Here's how the part is built. I have some questions about the finished solid (model axes, mm). Face numbers are marked on the shaded views. A direction names the side the tool comes from. Coordinates: 2 decimals unless noted, no trailing zeros. Loops run counter-clockwise (first coordinate to the right, second up) from the corner with the lowest first, then second, coordinate; pieces in that order, holes last. Notation, with made-up numbers: M 78.5,-29 L 109.5,-29 A28 ccw 109.5,-2 Z; hole C 25.5,-18.5 d3. An arc over 180 degrees is marked long. Use one line per item in the form item = value. Start each with the question number.
(1) Will these pins go through, and if not, where does the flat tip stop? P1, Ø6, axis at x = 18.5, z = 10.5, coming from the -Y side; P2, Ø2, axis at y = -5.5, z = 6.5, coming from the +X side; P3, Ø10, axis at x = 16.5, z = 9, coming from the +Y side.
(2) Imagine slicing it at A-A, the plane z = 10.25. Please give me the cut outline in (x, y).
(3) Please list where these lines run through material, in increasing order: L1, parallel to Y at x = 14, z = 13; L2, parallel to Z at x = 42, y = 3.5; L3, parallel to Z at x = 49.5, y = -3.75.
(4) Imagine slicing it at C-C, the plane x = 16.5. Please give me the cut outline in (y, z), and give its area (3 significant figures).
(5) Imagine slicing it at D-D, the plane z = 18.75. Please give me the cut outline in (x, y).
(6) On a 3-axis mill with a long thin cutter (end or side, diameter ignored), from which of +Z, -Z, +X, -X, +Y, -Y can I reach the whole of each face in a straight line? I mean the marked faces 1, 2, 3, 4 and 5. Say none if no direction works.
(7) Imagine slicing it at B-B, the plane y = 2.75. Please give me the cut outline in (x, z), and give its area (3 significant figures).
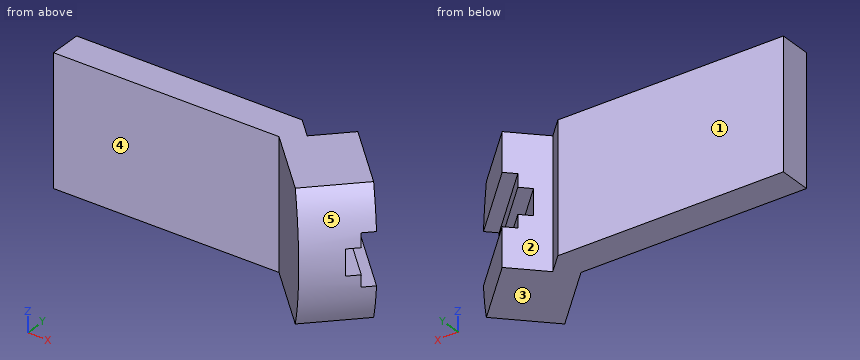
```python
from build123d import *

# Parameters (mm, degrees)
BOSS_EXTRUDE1_DEPTH      = 20
CUT_EXTRUDE5_DEPTH       = 6
CUT_EXTRUDE5_DEPTH_BACK  = 45.944197614
CUT_EXTRUDE10_DEPTH      = 8.5
CUT_EXTRUDE10_DEPTH_BACK = 43.444197614


with BuildPart() as part:
    # Sketch2 → Boss-Extrude1 (new body)
    with BuildSketch(Plane.XY):
        Polygon((0, 0), (35, 0), (45.883024287, -10.883024287), (52.954092099, -3.811956475), (42.347490381, 6.794645243), (37.776422569, 2.223577431), (35, 5), (0, 5), align=None)
    extrude(amount=BOSS_EXTRUDE1_DEPTH)

    # Sketch3 → Cut-Extrude5 (cut, two sides)
    with BuildSketch(Plane(origin=(28.383024287, -28.383024287, 0), x_dir=(0, 0, -1), z_dir=(0.707106781, -0.707106781, 0))) as cut_extrude5_sk:
        Polygon((-14, 134.13575902), (-14, 34.748737342), (-14, 32.748737342), (-12, 32.748737342), (-12, 30.748737342), (-8, 30.748737342), (-8, 32.748737342), (-6, 32.748737342), (-6, 34.748737342), (-6, 134.13575902), (-6, 332.909802377), (-14, 332.909802377), align=None)
    extrude(amount=CUT_EXTRUDE5_DEPTH, mode=Mode.SUBTRACT)
    extrude(cut_extrude5_sk.sketch, amount=-CUT_EXTRUDE5_DEPTH_BACK, mode=Mode.SUBTRACT)

    # Sketch4 → Cut-Extrude10 (cut, two sides)
    with BuildSketch(Plane(origin=(24.571067812, 24.571067812, 0), x_dir=(0, 0, -1), z_dir=(0.707106781, 0.707106781, 0))) as cut_extrude10_sk:
        with BuildLine():
            Line((-109.647389073, 14.29777825), (-20, -37.460165963))
            ThreePointArc((-20, -37.460165963), (-10, -40.139657887), (0, -37.460165963))
            Line((0, -37.460165963), (89.647389073, 14.29777825))
            Line((89.647389073, 14.29777825), (89.647389073, -192.733998604))
            Line((89.647389073, -192.733998604), (-109.647389073, -192.733998604))
            Line((-109.647389073, -192.733998604), (-109.647389073, 14.29777825))
        make_face()
    extrude(amount=CUT_EXTRUDE10_DEPTH, mode=Mode.SUBTRACT)
    extrude(cut_extrude10_sk.sketch, amount=-CUT_EXTRUDE10_DEPTH_BACK, mode=Mode.SUBTRACT)


solid = part.part
```
Answer:
q1.P1 = 0
q1.P2 = 51.56
q1.P3 = 5
q2.outline = M 0,0 L 35,0 L 45.88,-10.88 L 50.12,-6.64 L 39.52,3.97 L 37.78,2.22 L 35,5 L 0,5 Z
q3.L1 = 0 to 5
q3.L2 = 0 to 8, 12 to 20
q3.L3 = 0.34 to 8, 12 to 19.66
q4.outline = M 0,0 L 5,0 L 5,20 L 0,20 Z
q4.area = 100 mm²
q5.outline = M 0,0 L 35,0 L 44.46,-9.46 L 51.53,-2.39 L 42.35,6.79 L 37.78,2.22 L 35,5 L 0,5 Z
q6.face_1 = +Z, -Z, -X, +Y
q6.face_2 = +Z, -Z, +Y
q6.face_3 = -Z, +X, -X, +Y, -Y
q6.face_4 = +Z, -Z, -X, -Y
q6.face_5 = +X, -Y
q7.outline = M 0,0 L 37.25,0 L 37.25,20 L 0,20 Z; M 38.3,0 L 46.39,0 L 46.39,6 L 43.56,6 L 43.56,8 L 40.74,8 L 40.74,12 L 43.56,12 L 43.56,14 L 46.39,14 L 46.39,20 L 38.3,20 Z
q7.area = 873 mm²
